Could you check a few things on this model? Use its own coordinates, in mm. Face numbers are marked on the shaded views. Give positions to 0.01 mm unless a question says otherwise; leave off trailing zeros. Loops run counter-clockwise (first coordinate to the right, second up) from the corner with the lowest first, then second, coordinate; pieces in that order, holes last. Notation, with made-up numbers: M 85.25,26 L 127.25,26 A27 ccw 127.25,63 Z; hole C -7.75,8.25 d3. An arc over 180 degrees is marked long. Answer in a Markdown table with one row per item. Add a question column.
1. If we section it at A-A on z = 5: Count the separate pieces of the cut face and the enclosed holes in it, then the cut area to 3 significant figures.
2. I'm going to push flat-ended pins straight in: pin 1 Ø6 at (x, y) = (28, 8.5) entering from -Z; pin 2 Ø4 at (y, z) = (5, 5) entering from -X. Where does each tip first touch, or does it pass through?
3. If we section it at C-C on z = 8.25: List the corners of the cut face in (x, y) for me, then the cut area to 3 significant figures.
4. Thinking about a two-plate mould opening in Y: for the marked faces 1 and 2, which applies, released by +Y, released by -Y, zero draft, split by the parting line, or undercut?
5. I need wall thicknesses on line 1 along X through (y, z) = (7.5, 6); line 2 along X through (y, z) = (3, 3); line 3 along Y through (x, z) = (83.5, 2.5). Which ranges of each line are inside material? Lowest first, please. Write a range as from..to.
6. If we section it at D-D on x = 59: List the corners of the cut face in (y, z) for me, then the cut area to 3 significant figures.
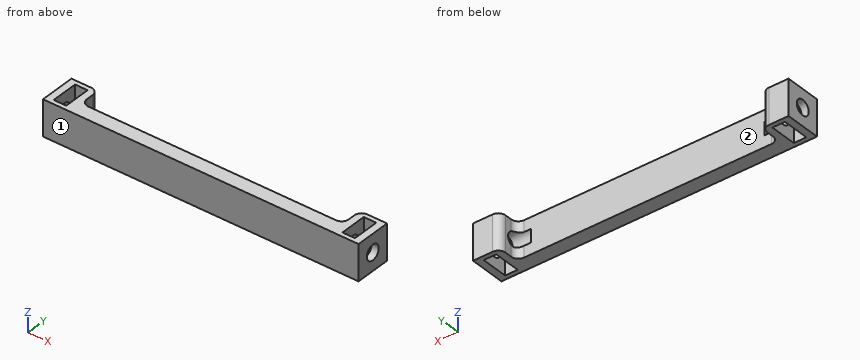
Autodesk Inventor part; units mm, degrees
ref_plane "Work Plane5" through (44.1, 0, 0) normal (1, 0, 0) x (0, 0, -1)
ref_plane "YZ Plane" through (0, 0, 0) normal (1, 0, 0) x (0, 1, 0)
ref_plane "XZ Plane" through (0, 0, 0) normal (0, 1, 0) x (-1, 0, 0)
sketch "Sketch11" plane through (0, 0, 0) normal (1, 0, 0) x (0, 1, 0)
  line L0 (0, 0) -> (10, 0)
  line L1 (10, 0) -> (10, 10)
  line L2 (10, 10) -> (0, 10)
  line L3 (0, 10) -> (0, 0)
  dimension "d27" = 10
  dimension "d28" = 10
extrude "Extrusion8" add sketch "Sketch11" along normal blind 88.2
sketch "Sketch12" plane through (0, 0, 0) normal (-1, 0, 0) x (0, 0, 1)
  circle A0 centre (5, 5) radius 2.1
  dimension "d31" = 4.2
extrude "Extrusion9" cut sketch "Sketch12" against normal blind 88.2
sketch "Sketch13" plane through (0, 0, 10) normal (0, 0, 1) x (1, 0, 0)
  line L0 (0, 10) -> (0, 0)
  line L1 (0, 10) -> (88.2, 10)
  line L2 (10, 10) -> (78.2, 10)
  line L3 (78.2, 10) -> (78.2, 4)
  line L4 (78.2, 4) -> (10, 4)
  line L5 (10, 4) -> (10, 10)
  dimension "d34" = 68.2
  dimension "d35" = 6
  dimension "d36" = 10
extrude "Extrusion10" cut sketch "Sketch13" against normal blind 88.2
sketch "Sketch14" plane through (0, 0, 10) normal (0, 0, 1) x (1, 0, 0)
  line L0 (0, 10) -> (10, 10)
  line L1 (0, 10) -> (0, 0)
  line L2 (2, 8.75) -> (5.5, 8.75)
  line L3 (5.5, 8.75) -> (5.5, 1.25)
  line L4 (5.5, 1.25) -> (2, 1.25)
  line L5 (2, 1.25) -> (2, 8.75)
  line L6 (10, 10) -> (7.5, 10)
  line L7 (7.5, 10) -> (7.5, 4)
  line L8 (7.5, 4) -> (10, 4)
  line L9 (10, 4) -> (10, 10)
  dimension "d39" = 3.5
  dimension "d40" = 7.5
  dimension "d41" = 1.25
  dimension "d42" = 2
  dimension "d43" = 2
extrude "Extrusion11" cut sketch "Sketch14" against normal blind 88.2
ref_plane "Work Plane5" through (44.1, 0, 0) normal (1, 0, 0) x (0, 0, -1)
mirror "Mirror4" about plane through (44.1, 0, 0) normal (1, 0, 0) of "Extrusion11", "Extrusion10"
sketch "Sketch15" plane through (7.5, 4, 3.1534) normal (0, 1, 0) x (1, 0, 0)
  line L0 (0, 0) -> (0, 3.1534)
  line L1 (4, 1.5767) -> (69.2, 1.5767)
  line L2 (69.2, 1.5767) -> (69.2, -5.2793)
  line L3 (69.2, -5.2793) -> (4, -5.2793)
  line L4 (4, -5.2793) -> (4, 1.5767)
  point P0 (-7.5, 3.1534)
  dimension "d47" = 65.2
  dimension "d48" = 4
extrude "Extrusion12" add sketch "Sketch15" against normal blind 3
fillet "Fillet2" radius 2 6 edges at (80.7, 10, 5) (80.7, 4, 8.4233) (80.7, 4, 1.5767) (7.5, 4, 1.5767) (7.5, 4, 8.4233) (7.5, 10, 5)
properties part number "BaseSlat"
Results:
| question | item | result |
|---|---|---|
| 1 | separate pieces | 3 |
| 1 | enclosed holes | 0 |
| 1 | area | 346 mm2 |
| 2 | pin 1 | through |
| 2 | pin 2 | x = 11.5 |
| 3 | outline | M 0,0 L 88.2,0 L 88.2,10 L 82.7,10 A2 ccw 80.7,8 L 80.7,6 A2 cw 78.7,4 L 9.5,4 A2 cw 7.5,6 L 7.5,8 A2 ccw 5.5,10 L 0,10 Z; hole M 2,1.25 L 5.5,1.25 L 5.5,8.75 L 2,8.75 Z; hole M 82.7,1.25 L 86.2,1.25 L 86.2,8.75 L 82.7,8.75 Z |
| 3 | area | 390 mm2 |
| 4 | face 1 | released by -Y |
| 4 | face 2 | released by +Y |
| 5 | line 1 | 0..2, 5.5..7.5, 80.7..82.7, 86.2..88.2 |
| 5 | line 2 | 0..2, 5.5..82.7, 86.2..88.2 |
| 5 | line 3 | 0..1.25, 8.75..10 |
| 6 | outline | M 0,0 L 4,0 L 4,10 L 0,10 Z |
| 6 | area | 40.0 mm2 |
